```python
from build123d import *

# Parameters (mm, degrees)
SKETCH1_W                         = 5
SKETCH1_H                         = 8
BOSS_EXTRUDE1_DEPTH               = 185
SKETCH2_R                         = 1
CUT_EXTRUDE2_DEPTH                = 2
F_2_0_2_DIAMETER_HOLE1_AT_2_COUNT = 2
F_2_0_2_DIAMETER_HOLE1_AT_2_PITCH = 20
LPATTERN1_COUNT                   = 8
LPATTERN1_PITCH                   = 20
SKETCH6_R                         = 1
CUT_EXTRUDE3_DEPTH                = 186.189767536
SKETCH8_R                         = 1.9
CUT_EXTRUDE4_DEPTH                = 2
SKETCH9_W                         = 5
SKETCH9_H                         = 8
CUT_EXTRUDE5_DEPTH                = 5


with BuildPart() as part:
    # Sketch1 → Boss-Extrude1 (new body)
    with BuildSketch(Plane.XY):
        Rectangle(SKETCH1_W, SKETCH1_H)
    extrude(amount=BOSS_EXTRUDE1_DEPTH)

    # Sketch2 → Cut-Extrude2 (cut)
    with BuildSketch(Plane(origin=(0, 4, 0), x_dir=(1, 0, 0), z_dir=(0, 1, 0))):
        with Locations(Location((0, -20, 0), (0, 0, 270))):
            Circle(SKETCH2_R)
        with Locations(Location((0, -40, 0), (0, 0, 270))):
            Circle(SKETCH2_R)
        with Locations(Location((0, -60, 0), (0, 0, 270))):
            Circle(SKETCH2_R)
        with Locations(Location((0, -80, 0), (0, 0, 270))):
            Circle(SKETCH2_R)
        with Locations(Location((0, -100, 0), (0, 0, 270))):
            Circle(SKETCH2_R)
        with Locations(Location((0, -120, 0), (0, 0, 270))):
            Circle(SKETCH2_R)
        with Locations(Location((0, -140, 0), (0, 0, 270))):
            Circle(SKETCH2_R)
        with Locations(Location((0, -160, 0), (0, 0, 270))):
            Circle(SKETCH2_R)
        with Locations(Location((0, -180, 0), (0, 0, 270))):
            Circle(SKETCH2_R)
    extrude(amount=-CUT_EXTRUDE2_DEPTH, mode=Mode.SUBTRACT)

    # Sketch4 → Ø2.0 (2) Diameter Hole1 (revolve, cut)
    with BuildSketch(Plane(origin=(0, 4, 20), x_dir=(0, 0, 1), z_dir=(1, 0, 0))):
        Polygon((0, 0), (0, 2.600860619), (1, 2), (1, 0), align=None)
    f_2_0_2_diameter_hole1 = revolve(axis=Axis((0, 10.35, 20), (0, -1, 0)), mode=Mode.SUBTRACT)

    # Ø2.0 (2) Diameter Hole1 at 2: Ø2.0 (2) Diameter Hole1 ×2
    with Locations(*[(0, 0, i * F_2_0_2_DIAMETER_HOLE1_AT_2_PITCH) for i in range(1, F_2_0_2_DIAMETER_HOLE1_AT_2_COUNT)]):
        add(f_2_0_2_diameter_hole1, mode=Mode.SUBTRACT)

    # LPattern1: Ø2.0 (2) Diameter Hole1 ×8
    with Locations(*[(0, 0, i * LPATTERN1_PITCH) for i in range(1, LPATTERN1_COUNT)]):
        add(f_2_0_2_diameter_hole1, mode=Mode.SUBTRACT)

    # LPattern1 copy 1 sketch → LPattern1 copy 1 (revolve, cut)
    with BuildSketch(Plane(origin=(0, 4, 60), x_dir=(0, 0, 1), z_dir=(1, 0, 0))):
        Polygon((0, 0), (0, 2.600860619), (1, 2), (1, 0), align=None)
    revolve(axis=Axis((0, 10.35, 60), (0, -1, 0)), mode=Mode.SUBTRACT)

    # LPattern1 copy 2 sketch → LPattern1 copy 2 (revolve, cut)
    with BuildSketch(Plane(origin=(0, 4, 80), x_dir=(0, 0, 1), z_dir=(1, 0, 0))):
        Polygon((0, 0), (0, 2.600860619), (1, 2), (1, 0), align=None)
    revolve(axis=Axis((0, 10.35, 80), (0, -1, 0)), mode=Mode.SUBTRACT)

    # LPattern1 copy 3 sketch → LPattern1 copy 3 (revolve, cut)
    with BuildSketch(Plane(origin=(0, 4, 100), x_dir=(0, 0, 1), z_dir=(1, 0, 0))):
        Polygon((0, 0), (0, 2.600860619), (1, 2), (1, 0), align=None)
    revolve(axis=Axis((0, 10.35, 100), (0, -1, 0)), mode=Mode.SUBTRACT)

    # LPattern1 copy 4 sketch → LPattern1 copy 4 (revolve, cut)
    with BuildSketch(Plane(origin=(0, 4, 120), x_dir=(0, 0, 1), z_dir=(1, 0, 0))):
        Polygon((0, 0), (0, 2.600860619), (1, 2), (1, 0), align=None)
    revolve(axis=Axis((0, 10.35, 120), (0, -1, 0)), mode=Mode.SUBTRACT)

    # LPattern1 copy 5 sketch → LPattern1 copy 5 (revolve, cut)
    with BuildSketch(Plane(origin=(0, 4, 140), x_dir=(0, 0, 1), z_dir=(1, 0, 0))):
        Polygon((0, 0), (0, 2.600860619), (1, 2), (1, 0), align=None)
    revolve(axis=Axis((0, 10.35, 140), (0, -1, 0)), mode=Mode.SUBTRACT)

    # LPattern1 copy 6 sketch → LPattern1 copy 6 (revolve, cut)
    with BuildSketch(Plane(origin=(0, 4, 160), x_dir=(0, 0, 1), z_dir=(1, 0, 0))):
        Polygon((0, 0), (0, 2.600860619), (1, 2), (1, 0), align=None)
    revolve(axis=Axis((0, 10.35, 160), (0, -1, 0)), mode=Mode.SUBTRACT)

    # LPattern1 copy 7 sketch → LPattern1 copy 7 (revolve, cut)
    with BuildSketch(Plane(origin=(0, 4, 180), x_dir=(0, 0, 1), z_dir=(1, 0, 0))):
        Polygon((0, 0), (0, 2.600860619), (1, 2), (1, 0), align=None)
    revolve(axis=Axis((0, 10.35, 180), (0, -1, 0)), mode=Mode.SUBTRACT)

    # Sketch6 → Cut-Extrude3 (cut, through all)
    with BuildSketch(Plane(origin=(0, 4, 0), x_dir=(1, 0, 0), z_dir=(0, 1, 0))):
        with Locations(Location((0, -30, 0), (0, 0, 270))):
            Circle(SKETCH6_R)
        with Locations(Location((0, -50, 0), (0, 0, 270))):
            Circle(SKETCH6_R)
        with Locations(Location((0, -70, 0), (0, 0, 270))):
            Circle(SKETCH6_R)
        with Locations(Location((0, -90, 0), (0, 0, 270))):
            Circle(SKETCH6_R)
        with Locations(Location((0, -110, 0), (0, 0, 270))):
            Circle(SKETCH6_R)
        with Locations(Location((0, -130, 0), (0, 0, 270))):
            Circle(SKETCH6_R)
        with Locations(Location((0, -150, 0), (0, 0, 270))):
            Circle(SKETCH6_R)
        with Locations(Location((0, -170, 0), (0, 0, 270))):
            Circle(SKETCH6_R)
        with Locations((0, -190)):
            Circle(SKETCH6_R)
        with Locations(Location((0, -10, 0), (0, 0, 270))):
            Circle(SKETCH6_R)
    extrude(amount=-CUT_EXTRUDE3_DEPTH, mode=Mode.SUBTRACT)

    # Sketch8 → Cut-Extrude4 (cut)
    with BuildSketch(Plane(origin=(0, 4, 0), x_dir=(1, 0, 0), z_dir=(0, 1, 0))):
        with Locations(Location((0, -10, 0), (0, 0, 270))):
            Circle(SKETCH8_R)
        with Locations(Location((0, -30, 0), (0, 0, 270))):
            Circle(SKETCH8_R)
        with Locations(Location((0, -50, 0), (0, 0, 270))):
            Circle(SKETCH8_R)
        with Locations(Location((0, -70, 0), (0, 0, 270))):
            Circle(SKETCH8_R)
        with Locations(Location((0, -90, 0), (0, 0, 270))):
            Circle(SKETCH8_R)
        with Locations(Location((0, -110, 0), (0, 0, 270))):
            Circle(SKETCH8_R)
        with Locations(Location((0, -130, 0), (0, 0, 270))):
            Circle(SKETCH8_R)
        with Locations(Location((0, -150, 0), (0, 0, 270))):
            Circle(SKETCH8_R)
        with Locations(Location((0, -170, 0), (0, 0, 270))):
            Circle(SKETCH8_R)
        with Locations((0, -190)):
            Circle(SKETCH8_R)
    extrude(amount=-CUT_EXTRUDE4_DEPTH, mode=Mode.SUBTRACT)

    # Sketch9 → Cut-Extrude5 (cut)
    with BuildSketch(Plane(origin=(0, 0, 0), x_dir=(-1, 0, 0), z_dir=(0, 0, -1))):
        Rectangle(SKETCH9_W, SKETCH9_H)
    extrude(amount=-CUT_EXTRUDE5_DEPTH, mode=Mode.SUBTRACT)


solid = part.part
```
Here's how the part is built. I have some questions about the finished solid (model axes, mm). A direction names the side the tool comes from. Give positions to 0.01 mm unless a question says otherwise; leave off trailing zeros. Use CSV: the item, a comma, the result in double quotes. Start each with the question number.
Item 1: On a 3-axis mill with a long thin cutter (end or side, diameter ignored), from which of +Z, -Z, +X, -X, +Y, -Y can I reach the whole of each face in a straight line? I mean faces 4 (the flat face through (0, 0, 185)), 5 (the flat face through (-1, 2, 111)). Say none if no direction works.
Item 2: I'm going to push a flat-ended pin straight in: P1, Ø1.1, axis at x = -1, z = 9.5, coming from the +Y side. Where does the tip first touch, or does it pass through?
Item 3: Thinking about a two-plate mould opening in Z: for faces 1 (the flat face through (0, 0, 5)), 2 (the cylindrical face through (0.571, 3.014, 31.812)), 3 (the flat face through (2.5, 0, 94)), which applies, pulls with the +Z half, pulls with the -Z half, needs draft (parallel to the pull), parting line crosses it, or undercut?
Item 4: If I drill on probe 1 along X at (y, z) = (2.9, 160); probe 2 along Y at (x, z) = (0.6, 131); probe 3 along Y at (x, z) = (-0.2, 139.5), over which ranges is the centre line in solid material (lowest first)? Write a range as [from, to].
Item 5: Suppose I cut it at A-A (y = -2.75). Give the number of separate pieces and of enclosed holes in the cut face, and give its area (3 significant figures).
Answer block:
1,face 4,"+Z, +X, -X, +Y, -Y"
1,face 5,"+Y"
2,P1,"stops at y = 2"
3,face 1,"pulls with the -Z half"
3,face 2,"undercut"
3,face 3,"needs draft"
4,probe 1,"x = [-2.5, -1], [1, 2.5]"
4,probe 2,"y = [-4, 2]"
4,probe 3,"y = [-4, 1.72]"
5,separate pieces,"1"
5,enclosed holes,"9"
5,area,"872 mm^2"
